Could you check a few things on this model? Use its own coordinates, in mm. A direction names the side the tool comes from. Coordinates: 2 decimals unless noted, no trailing zeros. Write each loop counter-clockwise with the first axis right and the second up, starting at its lowest first coordinate (ties: lowest second). Pieces come first, ordered by that corner, then holes. Notation, with made-up numbers: (50, 44) - (93, 44) arc R12 cw to (93, 50) - close; hole circle Ø5 at (78, 11.25). An arc over 180 degrees is marked (long way). Answer as a JSON object with one key per item and string values. Group by question number.
1) If we section it at A-A (x = 3.75): Write out the boundary of the cut face in (y, z) (1 decimal), plus the area to 3 significant figures.
2) On a 3-axis mill with a long thin cutter (end or side, diameter ignored), from which of +Z, -Z, +X, -X, +Y, -Y can I reach the whole of each face in a straight line? I mean faces 5 (the flat face through (0, -1, 1)), 6 (the cylindrical face through (9.568, 0.966, -1.26)), 7 (the conical face through (2.025, -2.868, 4.996)). Say none if no direction works.
3) We'd pull the mould along X, two halves only. Please class faces 1 (the flat face through (0, -4.8, 2.8)), 2 (the cylindrical face through (4.504, 0.966, -1.26)), 3 (the conical face through (-2.025, 2.893, -4.982)), 4 (the conical face through (2.025, 2.868, -4.996)): released by +X, released by -X, zero draft, split by the parting line, or undercut.
4) Please list where these lines run through material, in increasing order: line 1 along Y through (x, z) = (6, 0); line 2 along Y through (x, z) = (8, 0); line 3 along Z through (x, y) = (-1, 3.25).
5) Will these pins go through, and if not, where does the flat tip stop? pin 1 Ø2 at (y, z) = (0, 1) entering from -X; pin 2 Ø2 at (x, y) = (-3.5, 1) entering from +Z; pin 3 Ø4 at (x, z) = (-2, -4) entering from -Y; pin 4 Ø6.5 at (y, z) = (0, 0) entering from +X.
6) If we section it at B-B (x = -4.5): Write out the boundary of the cut face in (y, z), plus the area to 3 significant figures.
```python
from build123d import *

# Parameters (mm, degrees)
HEX_START               = 10.715625
HEX_HT_DEPTH            = 2.143125
SKETCH2_R               = 5.1435
EXTRUDE_L4_DEPTH        = 8.5725
EXTRUDE_L4_DRAFT        = -1.783333333
SKETCH9_W               = 12.85875
SKETCH9_H               = 0.5969
SKETCH11_OUTSIDE_W      = 75.416
SKETCH11_OUTSIDE_H      = 77.136
SKETCH11_OUTSIDE_R      = 5.55625
CUT_EXTRUDE3_DEPTH      = 16.407203436
CUT_EXTRUDE3_DRAFT      = -60
SKETCH12_OUTSIDE_W      = 75.416
SKETCH12_OUTSIDE_H      = 77.136
SKETCH12_OUTSIDE_R      = 5.55625
CUT_EXTRUDE5_DEPTH      = 16.407203436
CUT_EXTRUDE5_DRAFT      = -60
SKETCH14_R              = 0.9906
CUT_EXTRUDE6_DEPTH      = 16.407203436
CUT_EXTRUDE6_DEPTH_BACK = 16.407203436
SKETCH19_R              = 3.60045
CUT_EXTRUDE7_DEPTH      = 10.715625
CHAMFER1_SIZE           = 0.257175


with BuildPart() as part:
    # Sketch8 → Hex ht (new, symmetric)
    with BuildSketch(Plane(origin=(-10.715625, 0, 0), x_dir=(0, 0, -1), z_dir=(1, 0, 0)).offset(HEX_START)):
        Polygon((0, 6.415804866), (-5.55625, 3.207902433), (-5.55625, -3.207902433), (0, -6.415804866), (5.55625, -3.207902433), (5.55625, 3.207902433), align=None)
    extrude(amount=HEX_HT_DEPTH, both=True)


with BuildPart() as body_2:
    # Sketch2 → Extrude L4 (with draft: the straight prism first)
    with BuildSketch(Plane(origin=(-2.143125, 0, 0), x_dir=(0, 0, -1), z_dir=(1, 0, 0))):
        Circle(SKETCH2_R)
    extrude(amount=-EXTRUDE_L4_DEPTH)
    # Extrude L4: the draft: its side faces are tilted about the plane it starts from
    extrude_l4_sides = [body_2.faces().sort_by_distance(p)[0] for p in [
        (-6.429375, 0, 5.1435),
    ]]
    draft(extrude_l4_sides, Plane(origin=(-2.143125, 0, 0), x_dir=(0, 0, -1), z_dir=(1, 0, 0)), EXTRUDE_L4_DRAFT)

    # Sketch6 → Cut-Revolve1 (revolve, cut)
    with BuildSketch(Plane.XY, mode=Mode.PRIVATE) as cut_revolve1_sk:
        Polygon((-9.987395966, -4.899267892), (-10.715625, -4.171038858), (-10.715625, -4.876594414), align=None)
    revolve(cut_revolve1_sk.sketch.rotate(Axis((-10.715625, 0, 0), (1, 0, 0)), 90), axis=Axis((-10.715625, 0, 0), (1, 0, 0)), mode=Mode.SUBTRACT)

    # Combine2: union part
    add(part.part)

    # Sketch9 → Revolve1 (revolve)
    with BuildSketch(Plane.XY, mode=Mode.PRIVATE) as revolve1_sk:
        with Locations((4.28625, 1.28905)):
            Rectangle(SKETCH9_W, SKETCH9_H)
    revolve(revolve1_sk.sketch.rotate(Axis((0, 0, 0), (1, 0, 0)), 90), axis=Axis((0, 0, 0), (1, 0, 0)))

    # Sketch13 → Revolve2 (revolve)
    with BuildSketch(Plane.XY, mode=Mode.PRIVATE) as revolve2_sk:
        Polygon((8.387291667, 1.5875), (6.799791667, 1.905), (6.799791667, 1.5875), align=None)
    revolve(revolve2_sk.sketch.rotate(Axis((-10.715625, 0, 0), (1, 0, 0)), 90), axis=Axis((-10.715625, 0, 0), (1, 0, 0)))

    # Sketch17 → Revolve3 (revolve)
    with BuildSketch(Plane.XY, mode=Mode.PRIVATE) as revolve3_sk:
        Polygon((-2.143125, 1.905), (-1.593198869, 1.5875), (-2.143125, 1.5875), align=None)
    revolve(revolve3_sk.sketch.rotate(Axis((-10.715625, 0, 0), (1, 0, 0)), 270), axis=Axis((-10.715625, 0, 0), (1, 0, 0)))


with BuildPart() as cut_extrude3_tool:
    # Sketch11 outside → Cut-Extrude3 (with draft: the straight prism first)
    with BuildSketch(Plane(origin=(2.143125, 0, 0), x_dir=(0, 0, -1), z_dir=(1, 0, 0))):
        Rectangle(SKETCH11_OUTSIDE_W, SKETCH11_OUTSIDE_H)
        Circle(SKETCH11_OUTSIDE_R, mode=Mode.SUBTRACT)
    extrude(amount=-CUT_EXTRUDE3_DEPTH)
    # Cut-Extrude3: the draft: its side faces are tilted about the plane it starts from
    cut_extrude3_sides = [cut_extrude3_tool.faces().sort_by_distance(p)[0] for p in [
        (-6.060476718, -38.568, 0),
        (-6.060476718, 0, -37.708),
        (-6.060476718, 38.568, 0),
        (-6.060476718, 0, 37.708),
        (-6.060476718, 0, 5.55625),
    ]]
    draft(cut_extrude3_sides, Plane(origin=(2.143125, 0, 0), x_dir=(0, 0, -1), z_dir=(1, 0, 0)), CUT_EXTRUDE3_DRAFT)


with BuildPart() as body_2_1:
    add(body_2.part)

    # Cut-Extrude3: cut by cut_extrude3_tool
    add(cut_extrude3_tool.part, mode=Mode.SUBTRACT)


with BuildPart() as cut_extrude5_tool:
    # Sketch12 outside → Cut-Extrude5 (with draft: the straight prism first)
    with BuildSketch(Plane.ZY.offset(2.143125)):
        Rectangle(SKETCH12_OUTSIDE_W, SKETCH12_OUTSIDE_H)
        Circle(SKETCH12_OUTSIDE_R, mode=Mode.SUBTRACT)
    extrude(amount=-CUT_EXTRUDE5_DEPTH)
    # Cut-Extrude5: the draft: its side faces are tilted about the plane it starts from
    cut_extrude5_sides = [cut_extrude5_tool.faces().sort_by_distance(p)[0] for p in [
        (6.060476718, -38.568, 0),
        (6.060476718, 0, 37.708),
        (6.060476718, 38.568, 0),
        (6.060476718, 0, -37.708),
        (6.060476718, 0, -5.55625),
    ]]
    draft(cut_extrude5_sides, Plane.ZY.offset(2.143125), CUT_EXTRUDE5_DRAFT)


with BuildPart() as body_2_2:
    add(body_2_1.part)

    # Cut-Extrude5: cut by cut_extrude5_tool
    add(cut_extrude5_tool.part, mode=Mode.SUBTRACT)

    # Sketch14 → Cut-Extrude6 (cut, two sides)
    with BuildSketch(Plane.ZY.offset(2.143125)) as cut_extrude6_sk:
        Circle(SKETCH14_R)
    extrude(amount=CUT_EXTRUDE6_DEPTH, mode=Mode.SUBTRACT)
    extrude(cut_extrude6_sk.sketch, amount=-CUT_EXTRUDE6_DEPTH_BACK, mode=Mode.SUBTRACT)

    # Sketch19 → Cut-Extrude7 (cut)
    with BuildSketch(Plane.ZY.offset(10.715625)):
        Circle(SKETCH19_R)
    extrude(amount=-CUT_EXTRUDE7_DEPTH, mode=Mode.SUBTRACT)

    # Chamfer1
    chamfer1_edges = [body_2_2.edges().sort_by_distance(p)[0] for p in [
        (-10.715625, 0, -3.60045),
    ]]
    chamfer(chamfer1_edges, length=CHAMFER1_SIZE)


solid = body_2_2.part
```
Here are the results:
{
 "1": {"outline": "circle Ø3.2 at (0, 0); hole circle Ø2 at (0, 0)", "area": "4.83 mm²"},
 "2": {"face 5": "-X", "face 6": "+X", "face 7": "+Z, +X, -Y"},
 "3": {"face 1": "zero draft", "face 2": "undercut", "face 3": "released by -X", "face 4": "released by +X"},
 "4": {"line 1": "y = -1.59 to -0.99, 0.99 to 1.59", "line 2": "y = -1.66 to -0.99, 0.99 to 1.66", "line 3": "z = -5.48 to -1.55, 1.55 to 5.48"},
 "5": {"pin 1": "stops at x = 0", "pin 2": "stops at z = 5.12", "pin 3": "stops at y = -5.26", "pin 4": "stops at x = 10.72"},
 "6": {"outline": "circle Ø10.14 at (0, 0); hole circle Ø7.2 at (0, 0)", "area": "40.0 mm²"}
}
